Read the model definition and answer for the solid it produces. Units are mm, in the model's axes. Face numbers are marked on the shaded views. A direction names the side the tool comes from. Round coordinates to 2 decimals unless told otherwise and drop trailing zeros. Order: outer loops, then holes, each group sorted by start corner. A loop starts at its lowest first (then second) coordinate and runs counter-clockwise, first axis right, second up. Notation, with made-up numbers: (-26, -14.5) - (-20, -14.5) arc R23 cw to (-20, 21.5) - close; hole circle Ø5 at (71, -38). An arc over 180 degrees is marked (long way). Put each result on its own line as item: value. Start each with the question number.
Q1. For a pull along X with two mould halves and no side action, classify the marked faces 1, 2, 3 and 4 as pulls with the +X half, pulls with the -X half, needs draft (parallel to the pull), parting line crosses it, or undercut.
Q2. Find the intervals of material crossed by line 1 along Y through (x, z) = (26.5, 1); line 2 along Y through (x, z) = (-29, 19); line 3 along X through (y, z) = (25, -9), in increasing order. Write a range as from..to.
Q3. Section D-D on x = -10 is taken. Give the vertices of the cut face in (y, z), then the cut area to 3 significant figures.
Q4. Section C-C on z = -11 is taken. State how many separate pieces and enclosed holes the cut face has, then the cut area to 3 significant figures.
Q5. Section A-A on y = -36.83 is taken. Give the vertices of the cut face in (x, z), then the cut area to 3 significant figures.
Q6. Section B-B on y = 56 is taken. Give the vertices of the cut face in (x, z).
Q7. Which of the six approach directions +Z, -Z, +X, -X, +Y, -Y give full straight-line access (tool end or side, diameter ignored) to the marked faces 5 and 6?
Q8. This flat-tipped pin is pushed along its axis until it touches: pin 1 Ø18.5 at (x, y) = (-8, -16.5) entering from +Z. Where does it stop, or does it pass through?
from build123d import *

# Parameters (mm, degrees)
F1_DEPTH = 63.5
F3_DEPTH = 63.501
F4_W     = 3.9878
F4_H     = 2.032
F5_DEPTH = 63.5
F7_DEPTH = 63.501


with BuildPart() as f1:
    # F0 (on Front) → F1 (new body, symmetric)
    with BuildSketch(Plane.XZ):
        Polygon((31.75, -31.75), (31.75, 31.75), (25.4, 31.75), (25.4, -24.7142), (-25.4, -24.7142), (-25.4, 31.75), (-31.75, 31.75), (-31.75, -31.75), align=None)
    extrude(amount=F1_DEPTH, both=True)

    # F2 (on face) → F3 (cut, through all)
    with BuildSketch(Plane.YZ.offset(31.75)):
        with BuildLine():
            ThreePointArc((-59.436, 12.7), (-54.61, 7.874), (-49.784, 12.7))
            ThreePointArc((-49.784, 12.7), (-54.61, 17.526), (-59.436, 12.7))
        make_face()
        with BuildLine():
            Line((-49.784, -19.05), (-49.784, 12.7))
            ThreePointArc((-49.784, 12.7), (-54.61, 7.874), (-59.436, 12.7))
            Line((-59.436, 12.7), (-59.436, -19.05))
            ThreePointArc((-59.436, -19.05), (-54.61, -14.224), (-49.784, -19.05))
        make_face()
        with BuildLine():
            ThreePointArc((-59.436, -19.05), (-54.61, -23.876), (-49.784, -19.05))
            ThreePointArc((-49.784, -19.05), (-54.61, -14.224), (-59.436, -19.05))
        make_face()
        with BuildLine():
            ThreePointArc((-41.656, 12.7), (-36.83, 7.874), (-32.004, 12.7))
            ThreePointArc((-32.004, 12.7), (-36.83, 17.526), (-41.656, 12.7))
        make_face()
        with BuildLine():
            Line((-32.004, -19.05), (-32.004, 12.7))
            ThreePointArc((-32.004, 12.7), (-36.83, 7.874), (-41.656, 12.7))
            Line((-41.656, 12.7), (-41.656, -19.05))
            ThreePointArc((-41.656, -19.05), (-36.83, -14.224), (-32.004, -19.05))
        make_face()
        with BuildLine():
            ThreePointArc((-41.656, -19.05), (-36.83, -23.876), (-32.004, -19.05))
            ThreePointArc((-32.004, -19.05), (-36.83, -14.224), (-41.656, -19.05))
        make_face()
    extrude(amount=-F3_DEPTH, mode=Mode.SUBTRACT)

    # F4 (on Front) → F5 (cut, symmetric)
    with BuildSketch(Plane.XZ):
        with Locations((0, -25.7302)):
            Rectangle(F4_W, F4_H)
    extrude(amount=F5_DEPTH, both=True, mode=Mode.SUBTRACT)

    # F6 (on face) → F7 (cut, through all)
    with BuildSketch(Plane.YZ.offset(31.75)):
        with BuildLine():
            ThreePointArc((-28.956, -19.05), (-24.13, -23.876), (-19.304, -19.05))
            ThreePointArc((-19.304, -19.05), (-24.13, -14.224), (-28.956, -19.05))
        make_face()
        with BuildLine():
            ThreePointArc((-16.51, -19.05), (-11.684, -23.876), (-6.858, -19.05))
            ThreePointArc((-6.858, -19.05), (-11.684, -14.224), (-16.51, -19.05))
        make_face()
        with BuildLine():
            ThreePointArc((-28.956, -19.05), (-24.13, -14.224), (-19.304, -19.05))
            Line((-19.304, -19.05), (-19.304, 31.75))
            Line((-19.304, 31.75), (-28.956, 31.75))
            Line((-28.956, 31.75), (-28.956, -19.05))
        make_face()
        with BuildLine():
            Line((-6.858, 31.75), (-16.51, 31.75))
            Line((-16.51, 31.75), (-16.51, -19.05))
            ThreePointArc((-16.51, -19.05), (-11.684, -14.224), (-6.858, -19.05))
            Line((-6.858, -19.05), (-6.858, 31.75))
        make_face()
    extrude(amount=-F7_DEPTH, mode=Mode.SUBTRACT)


solid = f1.part
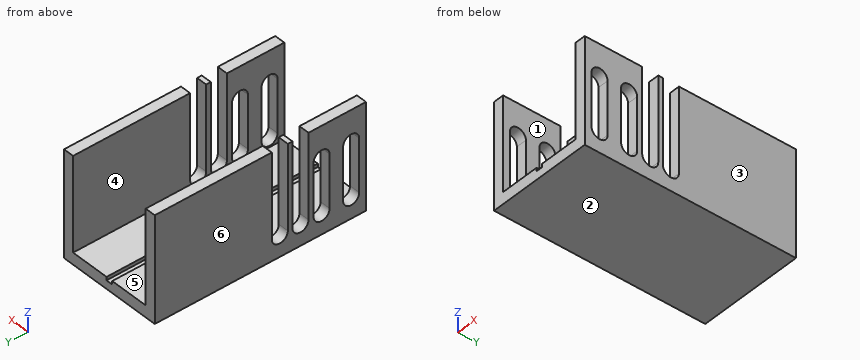
Findings:
1. face 1: undercut
1. face 2: needs draft
1. face 3: pulls with the +X half
1. face 4: undercut
2. line 1: -63.5..-59.44, -49.78..-41.66, -32..-28.96, -19.3..-16.51, -6.86..63.5
2. line 2: -63.5..-28.96, -19.3..-16.51, -6.86..63.5
2. line 3: -31.75..-25.4, 25.4..31.75
3. outline: (-63.5, -31.75) - (63.5, -31.75) - (63.5, -24.71) - (-63.5, -24.71) - close
3. area: 894 mm2
4. separate pieces: 10
4. enclosed holes: 0
4. area: 1,120 mm2
5. outline: (-31.75, -31.75) - (31.75, -31.75) - (31.75, -23.88) - (25.4, -23.88) - (25.4, -24.71) - (1.99, -24.71) - (1.99, -26.75) - (-1.99, -26.75) - (-1.99, -24.71) - (-25.4, -24.71) - (-25.4, -23.88) - (-31.75, -23.88) - close; (-31.75, 17.53) - (-25.4, 17.53) - (-25.4, 31.75) - (-31.75, 31.75) - close; (25.4, 17.53) - (31.75, 17.53) - (31.75, 31.75) - (25.4, 31.75) - close
5. area: 630 mm2
6. outline: (-31.75, -31.75) - (31.75, -31.75) - (31.75, 31.75) - (25.4, 31.75) - (25.4, -24.71) - (1.99, -24.71) - (1.99, -26.75) - (-1.99, -26.75) - (-1.99, -24.71) - (-25.4, -24.71) - (-25.4, 31.75) - (-31.75, 31.75) - close
7. face 5: +Z, +Y, -Y
7. face 6: +Z, -Z, -X, +Y, -Y
8. pin 1: z = -24.71
